Check sheet for the modelled part. Datum: model origin and axes. Units: mm. A direction names the side the tool comes from. Give positions to 0.01 mm unless a question says otherwise; leave off trailing zeros. Loops run counter-clockwise (first coordinate to the right, second up) from the corner with the lowest first, then second, coordinate; pieces in that order, holes last. Notation, with made-up numbers: M 1.5,7.25 L 56.5,7.25 A15 ccw 56.5,29.25 Z; hole C 20,-4 d1. An arc over 180 degrees is marked long. Use one line per item in the form item = value.
from build123d import *

# Parameters (mm, degrees)
F1_DEPTH = 25.4
F2_R     = 6.91991
F3_DEPTH = 25.4
F4_R     = 5.08


with BuildPart() as f1:
    # F0 (on Front) → F1 (new body)
    with BuildSketch(Plane.XZ):
        Polygon((-74.833319, 51.980667), (-74.833319, 20.457085), (-34.958635, 18.300878), (-34.958635, 51.980667), align=None)
    extrude(amount=F1_DEPTH)

    # F2 (on face) → F3 (join)
    with BuildSketch(Plane.XY.offset(51.980667)):
        with Locations((-56.627482, -15.38695)):
            Circle(F2_R)
    extrude(amount=F3_DEPTH)

    # F4
    f4_edges = [f1.edges().sort_by_distance(p)[0] for p in [
        (-63.547392, -15.38695, 77.380667),
    ]]
    fillet(f4_edges, radius=F4_R)


solid = f1.part
1) Section check C-C (z = 60). Record the cut outline in (x, y).
Evaluation:
outline = C -56.63,-15.39 d13.84
2) Section check B-B (x = -49). Record the cut outline in (y, z), then the cut area to 3 significant figures.
Evaluation:
outline = M -25.4,19.06 L 0,19.06 L 0,51.98 L -25.4,51.98 Z
area = 836 mm^2
3) Scan lines: line 1 (X direction, y = -12.75, z = 69.5); line 2 (Z direction, x = -41.5, y = -10.75); line 3 (Z direction, x = -56, y = -15). Record each from-to range of solid material in increasing order.
Evaluation:
line_1 = -63.03 to -50.23
line_2 = 18.65 to 51.98
line_3 = 19.44 to 77.38
4) Set-up check for faces 1 (the face through (-63.54, -15.08, 62)), 2 (the face through (-55, -25.4, 35)): record each of +Z, -Z, +X, -X, +Y, -Y from which the full face is reachable in a straight line by a thin tool's end or side.
Evaluation:
face_1 = +Z
face_2 = +Z, -Z, +X, -X, -Y
5) Depth check by flat-ended pin: pin 1 Ø8 at (x, z) = (-68, 30) entering from +Y; pin 2 Ø8 at (x, y) = (-39.5, -4.5) entering from +Z; pin 3 Ø5 at (x, y) = (-59, -17.5) entering from -Z. Enter the tip coordinate at first touch or a pass-through.
Evaluation:
pin_1 = 0
pin_2 = 51.98
pin_3 = 19.47
6) Section check A-A (y = -5.5). Record the cut outline in (x, z), then the cut area to 3 significant figures.
Evaluation:
outline = M -74.83,20.46 L -34.96,18.3 L -34.96,51.98 L -74.83,51.98 Z
area = 1,300 mm^2
